```python
from build123d import *

# Parameters (mm, degrees)
F0_W        = 304.4815510511
F0_H        = 164.8949235678
F1_DEPTH    = 35.13393
F3_DEPTH    = 76.30524
F4_R        = 12.7
F5_DEPTH    = 164.8959236678
F6_T1_DEPTH = 291.8949235678
F6_T3_DEPTH = 431.4815510511


# Not quite as in the source:
# - a fillet or chamfer that OpenCascade refuses, or shapes differently, is made with other operations: its cross-section is extruded or revolved along the edge and cut away or added


with BuildPart() as f1:
    # F0 (on Top) → F1 (new body)
    with BuildSketch(Plane.XY):
        with Locations((1.1980161071, -3.480002284)):
            Rectangle(F0_W, F0_H)
    extrude(amount=F1_DEPTH)

    # F2 (on Right) → F3 (cut)
    with BuildSketch(Plane.YZ):
        with BuildLine():
            add(Edge.make_bspline(
                [(-153.2041430473, 84.2628479004), (-91.991528101, 80.6964321278), (-18.1249389438, 101.4390649478), (-6.3535316821, 35.464664407), (123.7363166686, 35.8483556733), (-7.6536515228, -20.5708818303), (-72.9342844873, 34.9796073045), (-103.3804491162, 54.5991994441)],
                knots=[0, 0, 0, 0, 0.2418010288, 0.3897431708, 0.5754176067, 0.7622533627, 1, 1, 1, 1], degree=3))
            add(Edge.make_bspline(
                [(-153.2041430473, 84.2628479004), (-136.2230330706, 76.9635861119), (-120.361559093, 61.8984612326), (-103.3804491162, 54.5991994441)],
                knots=[0, 0, 0, 0, 57.985623362, 57.985623362, 57.985623362, 57.985623362], degree=3))
        make_face()
    extrude(amount=-F3_DEPTH, mode=Mode.SUBTRACT)

    # F4 (on face) → F5 (cut, through all)
    with BuildSketch(Plane(origin=(0, 78.9674594998, 0), x_dir=(-1, 0, 0), z_dir=(0, 1, 0))):
        with Locations((-127, 0)):
            Circle(F4_R)
        with Locations((-76.2, 0)):
            Circle(F4_R)
        Circle(F4_R)
    extrude(amount=-F5_DEPTH, mode=Mode.SUBTRACT)

    # F6: fillet of radius 25.4 on 4 edges, made by hand

    # F6_s2 → F6_t1 (cut)
    with BuildSketch(Plane.XZ.offset(-142.4674594998)):
        with BuildLine():
            ThreePointArc((128.0387916327, 35.13393), (145.9993038748, 27.6944422421), (153.4387916327, 9.73393))
            Line((153.4387916327, 9.73393), (153.4387916327, 35.13393))
            Line((153.4387916327, 35.13393), (128.0387916327, 35.13393))
        make_face()
        with BuildLine():
            ThreePointArc((-151.0427594185, 9.73393), (-143.6032716606, 27.6944422421), (-125.6427594185, 35.13393))
            Line((-125.6427594185, 35.13393), (-151.0427594185, 35.13393))
            Line((-151.0427594185, 35.13393), (-151.0427594185, 9.73393))
        make_face()
    extrude(amount=F6_T1_DEPTH, mode=Mode.SUBTRACT)

    # F6_s4 → F6_t3 (cut)
    with BuildSketch(Plane.YZ.offset(-214.5427594185)):
        with BuildLine():
            ThreePointArc((78.9674594998, 9.73393), (71.527971742, 27.6944422421), (53.5674594998, 35.13393))
            Line((53.5674594998, 35.13393), (78.9674594998, 35.13393))
            Line((78.9674594998, 35.13393), (78.9674594998, 9.73393))
        make_face()
        with BuildLine():
            ThreePointArc((-60.5274640679, 35.13393), (-78.4879763101, 27.6944422421), (-85.9274640679, 9.73393))
            Line((-85.9274640679, 9.73393), (-85.9274640679, 35.13393))
            Line((-85.9274640679, 35.13393), (-60.5274640679, 35.13393))
        make_face()
    extrude(amount=F6_T3_DEPTH, mode=Mode.SUBTRACT)


solid = f1.part
```
Geometry: final body of the model. Coordinates: model frame, mm. A direction names the side the tool comes from. Coordinates: 2 decimals unless noted, no trailing zeros. Write each loop counter-clockwise with the first axis right and the second up, starting at its lowest first coordinate (ties: lowest second). Pieces come first, ordered by that corner, then holes. Notation, with made-up numbers: M 48,61.5 L 99,61.5 A19 ccw 99,97.5 Z; hole C 54.5,-33.5 d11. An arc over 180 degrees is marked long. Use CSV: the item, a comma, the result in double quotes. Start each with the question number.
1. Mould query, pull axis X, two halves, no side actions, for faces 1 (the face through (-101, -3, 35.134)), 2 (the face through (126.721, -2.326, 12.697)), 3 (the face through (-151.043, -5, 5)), 4 (the face through (145.8, -2.33, 27.89)). Classes: pulls with the +X half, pulls with the -X half, needs draft (parallel to the pull), parting line crosses it, or undercut.
2. Ray query, probe 1 along X at (y, z) = (9, 5); probe 2 along X at (y, z) = (-26, 11.5); probe 3 along X at (y, z) = (36.5, 31). Return the intervals inside material, ascending.
3. Cut plane B-B on x = 76.2. Return the cut outline in (y, z).
4. First-contact query: P1, Ø2, axis at x = -24, y = 44, coming from the +Z side; P2, Ø8, axis at x = -33, z = 19.5, coming from the +Y side; P3, Ø3, axis at x = 116, z = 26, coming from the +Y side. Flat tips, straight axial feed; report the tip coordinate or a pass-through.
5. Reachability of faces 5 (the face through (0, 4, 24)), 6 (the face through (153.439, -5, 5)) from +Z, -Z, +X, -X, +Y, -Y: full face, straight path, thin tool, end or side. Return the list, or none.
6. Cut plane A-A on x = 36.5. Return the cut outline in (y, z).
Entries:
1,face 1,"needs draft"
1,face 2,"undercut"
1,face 3,"pulls with the -X half"
1,face 4,"pulls with the +X half"
2,probe 1,"-151.04 to -76.31, 11.67 to 64.53, 87.87 to 115.33, 138.67 to 153.44"
2,probe 2,"-150.98 to -76.31, 5.39 to 70.81, 81.59 to 121.61, 132.39 to 153.38"
2,probe 3,"-139.53 to -76.31, 0 to 141.93"
3,outline,"M -85.75,12.7 L 78.79,12.7 A25.4 ccw 53.57,35.13 L -60.53,35.13 A25.4 ccw Z"
4,P1,"z = 6.92"
4,P2,"y = 78.3"
4,P3,"y = 74.23"
5,face 5,"+Z"
5,face 6,"+Z, -Z, +X, +Y, -Y"
6,outline,"M -85.93,0 L 78.97,0 L 78.97,9.73 A25.4 ccw 53.57,35.13 L -60.53,35.13 A25.4 ccw -85.93,9.73 Z"
